Could you check a few things on this model? Use its own coordinates, in mm. Give positions to 0.01 mm unless a question says otherwise; leave off trailing zeros. Loops run counter-clockwise (first coordinate to the right, second up) from the corner with the lowest first, then second, coordinate; pieces in that order, holes last. Notation, with made-up numbers: (62.25, 71) -> (71.25, 71) arc R14 cw to (71.25, 92) -> close; hole circle Ø7 at (43, -4.75). An arc over 180 degrees is marked (long way). Put each result on its own line as item: value.
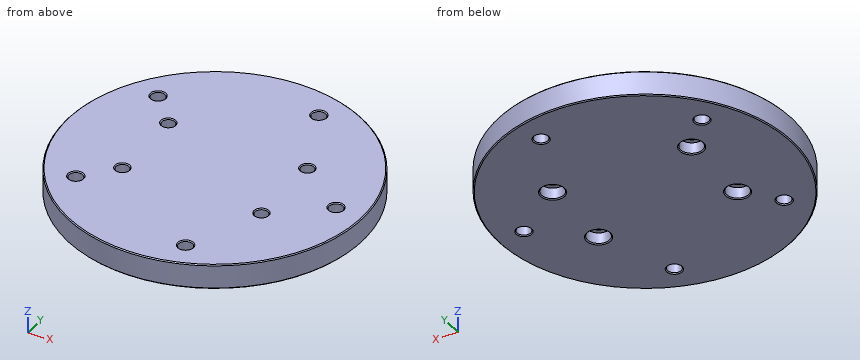
```python
from build123d import *

# Parameters (mm, degrees)
F0_R           = 75
F1_DEPTH       = 12.7
F2_D           = 6.6
F2_CBORE_D     = 11.25
F2_CBORE_DEPTH = 6
F4_D           = 7
F5_SIZE        = 0.5
F7_ANGLE       = -90


with BuildPart() as f1:
    # F0 (on Top) → F1 (new body)
    with BuildSketch(Plane.XY):
        Circle(F0_R)
    extrude(amount=F1_DEPTH)

    # F2 (through all)
    with Locations(Plane(origin=(0, 0, 0), x_dir=(1, 0, 0), z_dir=(0, 0, -1))):
        with Locations((-20, -35), (20, -35), (-20, 35), (20, 35)):
            CounterBoreHole(F2_D / 2, F2_CBORE_D / 2, F2_CBORE_DEPTH)

    # F4 (through all)
    with Locations(Plane.XY.offset(12.7)):
        with Locations((0, 61), (58, 18.8), (35.8, -49.3), (-35.8, -49.3), (-58, 18.8)):
            Hole(F4_D / 2)

    # F5
    f5_edges = [f1.edges().sort_by_distance(p)[0] for p in [
        (-75, 0, 12.7),
        (-39.3, -49.3, 12.7),
        (-23.3, -35, 12.7),
        (16.7, -35, 12.7),
        (32.3, -49.3, 12.7),
        (-61.5, 18.8, 12.7),
        (-23.3, 35, 12.7),
        (16.7, 35, 12.7),
        (54.5, 18.8, 12.7),
        (-3.5, 61, 12.7),
        (-75, 0, 0),
        (-39.3, -49.3, 0),
        (-25.625, -35, 0),
        (14.375, -35, 0),
        (32.3, -49.3, 0),
        (-61.5, 18.8, 0),
        (-25.625, 35, 0),
        (14.375, 35, 0),
        (54.5, 18.8, 0),
        (-3.5, 61, 0),
    ]]
    chamfer(f5_edges, length=F5_SIZE)


with BuildPart() as f1_1:
    # F7: moved
    add(f1.part.rotate(Axis((0, 0, 4.841263406), (0, 0, 1)), F7_ANGLE))


solid = f1_1.part
```
1. I need wall thicknesses on line 1 (X direction, y = 0, z = 6.5); line 2 (X direction, y = 20, z = 3.5) (3 decimals); line 3 (Y direction, x = 36, z = 11.25). Which ranges of each line are inside material? Lowest first, please.
Recorded:
line 1: x = -75 to 57.5, 64.5 to 75
line 2: x = -72.284 to -40.625, -29.375 to 29.375, 40.625 to 72.284
line 3: y = -65.8 to -23.14, -16.86 to 16.86, 23.14 to 65.8
2. If we section it at B-B (z = 3.5): Count the separate pieces of the cut face and the enclosed holes in it, then the cut area to 3 significant figures.
Recorded:
separate pieces: 1
enclosed holes: 9
area: 17,100 mm^2
3. If we section it at A-A (y = 0): List the corners of the cut face in (x, z) for me.
Recorded:
outline: (-75, 0.5) -> (-74.5, 0) -> (57, 0) -> (57.5, 0.5) -> (57.5, 12.2) -> (57, 12.7) -> (-74.5, 12.7) -> (-75, 12.2) -> close; (64.5, 0.5) -> (65, 0) -> (74.5, 0) -> (75, 0.5) -> (75, 12.2) -> (74.5, 12.7) -> (65, 12.7) -> (64.5, 12.2) -> close
4. I'm going to push flat-ended pins straight in: pin 1 (4 mm diameter, centred on y = 12.5, z = 8, fed in from -X); pin 2 (5.5 mm diameter, centred on x = 33.5, y = -19.5, fed in from -Z); pin 3 (6.5 mm diameter, centred on x = 18.8, y = -58, fed in from +Z); pin 4 (4 mm diameter, centred on x = -18, z = 5, fed in from +Y). Where does each tip first touch, or does it pass through?
Recorded:
pin 1: stops at x = -74.26
pin 2: stops at z = 6
pin 3: passes through
pin 4: stops at y = 73.27
